Autodesk Inventor part; units mm, degrees
ref_plane "YZ Plane" through (0, 0, 0) normal (1, 0, 0) x (0, 1, 0)
ref_plane "XZ Plane" through (0, 0, 0) normal (0, 1, 0) x (-1, 0, 0)
ref_plane "XY Plane" through (0, 0, 0) normal (0, 0, 1) x (1, 0, 0)
sketch "Эскиз1" plane through (0, 0, 0) normal (0, 1, 0) x (-1, 0, 0)
  line L0 (0, 0) -> (97.5, 0)
  line L1 (97.5, 0) -> (97.5, -9)
  line L2 (97.5, -9) -> (75, -9)
  line L3 (75, -9) -> (75, -15)
  line L4 (0, -4) -> (0, 0)
  line L5 (75, -15) -> (69, -15)
  line L6 (69, -15) -> (69, -4)
  line L7 (69, -4) -> (0, -4)
  dimension "d0" = 195
  dimension "d1" = 150
  dimension "d3" = 9
  dimension "d5" = 15
  dimension "d6" = 138
  dimension "d7" = 4
revolve "Вращение1" add sketch "Эскиз1" angle 360 about axis through (0, 0, -4) along (0, 0, 1)
sketch "Эскиз3" plane through (0, 0, 0) normal (0, 0, 1) x (1, 0, 0)
  circle A0 centre (0, 0) radius 86.25 construction
  line L0 (0, 0) -> (-91.162, -91.162) construction
  line L1 (0, 0) -> (128.9225, 0) construction
  point P0 (0, 0)
  point P1 (-60.988, -60.988)
  point P2 (60.988, -60.988)
  point P3 (60.988, 60.988)
  point P4 (-60.988, 60.988)
  dimension "d15" = 172.5
  dimension "d16" = 135
  dimension "d19" = 360
hole "Отверстие1" at (-60.988, -60.988, 0) at (60.988, -60.988, 0) at (60.988, 60.988, 0) at (-60.988, 60.988, 0) direction (0, 0, -1) diameter 8.376 end through all
chamfer "Фаска1" distance 2 angle 45 2 edges at (75, 0, -15) (97.5, 0, 0)
properties part number "МПСТ Крышка подшипника глухая 150" material "Сталь, углеродистая"
The model under review builds one solid part; all positions refer to its coordinate system, in mm. A direction names the side the tool comes from. Coordinates: 2 decimals unless noted, no trailing zeros. Write each loop counter-clockwise with the first axis right and the second up, starting at its lowest first coordinate (ties: lowest second). Pieces come first, ordered by that corner, then holes. Notation, with made-up numbers: (55, -34.5) -> (67, -34.5) arc R19 ccw to (67, 0.5) -> close; hole circle Ø10 at (-6, 70). An arc over 180 degrees is marked (long way). Answer in a Markdown table with one row per item.
1. Clearance check with flat-ended pins moving along their axes: pin 1 Ø1.5 at (y, z) = (67, -4) entering from -X; pin 2 Ø7.5 at (x, y) = (-60.988, -60.988) entering from -Z; pin 3 Ø5 at (x, z) = (-16.5, -12) entering from +Y; pin 4 Ø12 at (x, y) = (2.5, -39.5) entering from -Z. State where each tip first meets the part, or that it passes through.
Answers below:
| item | result |
|---|---|
| pin 1 | stops at x = -71.53 |
| pin 2 | passes through |
| pin 3 | stops at y = 73.68 |
| pin 4 | stops at z = -4 |
2. For faces 4 (the cylindrical face through (-65.14, 61.53, -4.56)), 5 (the flat face through (1, -1, -4)), list the 3-axis set-ups (+Z, -Z, +X, -X, +Y, -Y) from which the entire face can be reached by the end or side of a thin tool; tool diameter is ignored.
Answers below:
| item | result |
|---|---|
| face 4 | +Z, -Z |
| face 5 | -Z |
3. Wall thickness on probe 1 along Z at (x, y) = (14, -67); probe 2 along Z at (x, y) = (-25.5, -80); probe 3 along X at (y, z) = (0, -7.25): over which ranges is each line inside the solid? List them lowest first. Write a range as [from, to].
Answers below:
| item | result |
|---|---|
| probe 1 | z = [-4, 0] |
| probe 2 | z = [-9, 0] |
| probe 3 | x = [-97.5, -69], [69, 97.5] |
4. Draft analysis for pull direction Y (two halves, no side actions). For faces 1 (the flat face through (-54, -44, -15)), 2 (the cylindrical face through (56.836, 61.533, -4.563)), 3 (the conical face through (-91.209, 28.723, -0.125)), state which applies: +Y half, -Y half, draft (parallel to the pull), parting line (faces both ways), or undercut.
Answers below:
| item | result |
|---|---|
| face 1 | draft |
| face 2 | undercut |
| face 3 | parting line |
5. We need section A-A, the plane y = 0. State the section outline as (x, z) points, and give its area (3 significant figures).
Answers below:
| item | result |
|---|---|
| outline | (-97.5, -9) -> (-75, -9) -> (-75, -13) -> (-73, -15) -> (-69, -15) -> (-69, -4) -> (69, -4) -> (69, -15) -> (73, -15) -> (75, -13) -> (75, -9) -> (97.5, -9) -> (97.5, -2) -> (95.5, 0) -> (-95.5, 0) -> (-97.5, -2) -> close |
| area | 1,130 mm^2 |
